Build history of the part. All positions in model axes, mm. Give positions to 0.01 mm unless a question says otherwise; leave off trailing zeros. Order: outer loops, then holes, each group sorted by start corner. A loop starts at its lowest first (then second) coordinate and runs counter-clockwise, first axis right, second up. Notation, with made-up numbers: (28, 40) -> (72, 40) arc R28 ccw to (72, 71) -> close; hole circle Ø10 at (-19, -33). An arc over 180 degrees is marked (long way). One line per question, with ' | ' between items. Start each with the question number.
(1) Drill centre lines: L1, parallel to X at y = 5.25, z = 0; L2, parallel to X at y = 8.5, z = 5 (3 decimals); L3, parallel to X at y = 7.25, z = -3. Where is each one in solid material? Low to high. Write a range as from..to.
(2) Pull direction Z, two halves, no side cores. Call faces 1 (the face through (-29, 5, 13)), 2 (the face through (-30, 5, 0)), 3 (the face through (0, 5, -15)), 4 (the face through (13.852, 4.93, 10.026)): +Z half, -Z half, draft (parallel to the pull), parting line (faces both ways), or undercut.
(3) Cut at B-B (x = -12.5). Give the cut face in (y, z), then the cut area to 3 significant figures.
(4) Cut at C-C (z = -11.5). Give the cut face in (x, y), then the cut area to 3 significant figures.
(5) Pin check, flat tip, straight feed: pin 1 Ø2.5 at (x, z) = (12.5, 11.5) entering from -Y. Stop position of the tip, or through.
(6) Cut at D-D (y = 6.75). Give the number of separate pieces and of enclosed holes in the cut face, then the cut area to 3 significant figures.
(7) Cut at A-A (x = 12.5). Give the cut face in (y, z), then the cut area to 3 significant figures.
from build123d import *

# Parameters (mm, degrees)
SKETCH1_W           = 60
SKETCH1_H           = 30
SKETCH1_R           = 8
SKETCH1_R_2         = 6
SKETCH1_R_3         = 1.75
SKETCH1_R_4         = 2
BOSS_EXTRUDE1_DEPTH = 10
FILLET1_R           = 5


with BuildPart() as part:
    # Sketch1 → Boss-Extrude1 (new body)
    with BuildSketch(Plane(origin=(0, 0, 0), x_dir=(1, 0, 0), z_dir=(0, 1, 0))):
        Rectangle(SKETCH1_W, SKETCH1_H)
        with Locations(Location((12.5, 0, 0), (0, 0, 270))):
            Circle(SKETCH1_R, mode=Mode.SUBTRACT)
        with Locations(Location((-12.5, 0, 0), (0, 0, 270))):
            Circle(SKETCH1_R_2, mode=Mode.SUBTRACT)
        with Locations(Location((-18.156854249, 5.656854249, 0), (0, 0, 270))):
            Circle(SKETCH1_R_3, mode=Mode.SUBTRACT)
        with Locations(Location((-6.843145751, 5.656854249, 0), (0, 0, 270))):
            Circle(SKETCH1_R_3, mode=Mode.SUBTRACT)
        with Locations(Location((-6.843145751, -5.656854249, 0), (0, 0, 270))):
            Circle(SKETCH1_R_3, mode=Mode.SUBTRACT)
        with Locations(Location((-18.156854249, -5.656854249, 0), (0, 0, 270))):
            Circle(SKETCH1_R_3, mode=Mode.SUBTRACT)
        with Locations(Location((12.5, -11.5, 0), (0, 0, 270))):
            Circle(SKETCH1_R_4, mode=Mode.SUBTRACT)
        with Locations(Location((12.5, 11.5, 0), (0, 0, 270))):
            Circle(SKETCH1_R_4, mode=Mode.SUBTRACT)
    extrude(amount=BOSS_EXTRUDE1_DEPTH)

    # Fillet1
    fillet1_edges = [part.edges().sort_by_distance(p)[0] for p in [
        (30, 5, 15),
        (-30, 5, 15),
        (-30, 5, -15),
        (30, 5, -15),
    ]]
    fillet(fillet1_edges, radius=FILLET1_R)


solid = part.part
Result set:
1) L1: x = -30..-18.5, -6.5..4.5, 20.5..30 | L2: x = -30..-19.779, -16.535..-15.817, -9.183..-8.465, -5.221..6.255, 18.745..30 | L3: x = -30..-17.7, -7.3..5.08, 19.92..30
2) face 1: +Z half | face 2: draft | face 3: -Z half | face 4: undercut
3) outline: (0, -15) -> (10, -15) -> (10, -6) -> (0, -6) -> close; (0, 6) -> (10, 6) -> (10, 15) -> (0, 15) -> close | area: 180 mm2
4) outline: (-29.77, 0) -> (10.5, 0) -> (10.5, 10) -> (-29.77, 10) -> close; (14.5, 0) -> (29.77, 0) -> (29.77, 10) -> (14.5, 10) -> close | area: 555 mm2
5) pin 1: passes through
6) separate pieces: 1 | enclosed holes: 8 | area: 1,400 mm2
7) outline: (0, -15) -> (10, -15) -> (10, -13.5) -> (0, -13.5) -> close; (0, -9.5) -> (10, -9.5) -> (10, -8) -> (0, -8) -> close; (0, 8) -> (10, 8) -> (10, 9.5) -> (0, 9.5) -> close; (0, 13.5) -> (10, 13.5) -> (10, 15) -> (0, 15) -> close | area: 60.0 mm2
